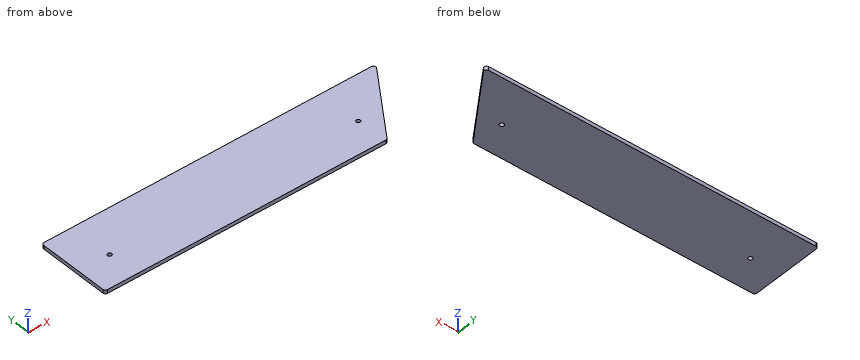
Autodesk Inventor part; units mm, degrees
ref_plane "YZ Plane" through (0, 0, 0) normal (1, 0, 0) x (0, 1, 0)
ref_plane "XZ Plane" through (0, 0, 0) normal (0, 1, 0) x (-1, 0, 0)
ref_plane "XY Plane" through (0, 0, 0) normal (0, 0, 1) x (1, 0, 0)
sketch "Sketch1" plane through (0, 0, 0) normal (0, 0, 1) x (1, 0, 0)
  line L0 (-134.5, -30) -> (134.5, -30)
  line L1 (134.5, -30) -> (134.5, 30)
  line L2 (134.5, 30) -> (-134.5, 30)
  line L3 (-134.5, 30) -> (-134.5, -30)
  line L4 (-134.5, -30) -> (134.5, 30) construction
  line L5 (134.5, -30) -> (-134.5, 30) construction
  line L6 (134.5, 30) -> (92.4875, -30)
  point P0 (0, 0)
  dimension "d0" = 269
  dimension "d1" = 60
  dimension "d2" = 55
extrude "Extrusion1" add sketch "Sketch1" along normal blind 3 contours L3 L2 L6 L0
sketch "Sketch2" plane through (0, 0, 3) normal (0, 0, 1) x (1, 0, 0)
  circle A0 centre (-109.5, -5) radius 1.65
  line L0 (-134.5, -30) -> (92.4875, -30)
  line L1 (-134.5, 30) -> (-134.5, -30)
  line L2 (-109.5, -5) -> (151.1099, -5) construction
  circle A1 centre (90.5, -5) radius 1.65
  point P0 (0, 0)
  dimension "d5" = 25
  dimension "d6" = 3.3
  dimension "d7" = 25
  dimension "d8" = 225
  dimension "d9" = 3.3
extrude "Extrusion2" cut sketch "Sketch2" against normal through all
fillet "Fillet1" radius 2 4 edges at (-134.5, 30, 1.5) (-134.5, -30, 1.5) (92.4875, -30, 1.5) (134.5, 30, 1.5)
sketch "Sketch3" plane through (0, 0, 3) normal (0, 0, 1) x (1, 0, 0)
  arc A0 (132.2963, 26.8528) -> (130.658, 30) centre (130.658, 28) ccw
  line L0 (130.658, 30) -> (-132.5, 30)
  arc A1 (-132.5, 30) -> (-134.5, 28) centre (-132.5, 28) ccw
  line L1 (-134.5, 28) -> (-134.5, -28)
  arc A2 (-134.5, -28) -> (-132.5, -30) centre (-132.5, -28) ccw
  line L2 (-132.5, -30) -> (91.4464, -30)
  arc A3 (91.4464, -30) -> (93.0847, -29.1472) centre (91.4464, -28) ccw
  line L3 (93.0847, -29.1472) -> (132.2963, 26.8528)
  circle A4 centre (90.5, -5) radius 1.65
  circle A5 centre (-109.5, -5) radius 1.65
  point P0 (0, 0)
equation "\"d9\" = d6"
properties part number "UpperAcrylicSheetSide"
The listing builds one solid part. Answer for the finished solid, in the listing's coordinates (mm). Coordinates: 2 decimals unless noted, no trailing zeros. Loops run counter-clockwise (first coordinate to the right, second up) from the corner with the lowest first, then second, coordinate; pieces in that order, holes last. Notation, with made-up numbers: (11, 26.5) -> (47, 26.5) arc R20 ccw to (47, 41.5) -> close; hole circle Ø3 at (-30.5, 43). An arc over 180 degrees is marked (long way). Answer in a Markdown table with one row per item. Add a question column.
1. The part is cut by section B-B, the plane y = -13. Write down the section's boundary in (x, z).
2. The part is cut by section C-C, the plane y = 14. Write down the section's boundary in (x, z).
3. A flat-ended cylindrical pin translates along its axis: P1, Ø1, axis at x = 97, z = 1, coming from the -Y side. Find the tip coordinate at first contact, or state that the pin passes through.
4. The part is cut by section A-A, the plane z = 1.3. Write down the section's boundary in (x, y), then the cut area to 3 significant figures.
5. Consider line 1 (Y direction, x = -109.5, z = 0.65); line 2 (X direction, y = -24.5, z = 0.5); line 3 (X direction, y = 8.5, z = 1.1). Determine where each line is inside the solid, lowest interval first. Write a range as [from, to].
Answer below:
| question | item | result |
|---|---|---|
| 1 | outline | (-134.5, 0) -> (104.39, 0) -> (104.39, 3) -> (-134.5, 3) -> close |
| 2 | outline | (-134.5, 0) -> (123.3, 0) -> (123.3, 3) -> (-134.5, 3) -> close |
| 3 | P1 | y = -24.27 |
| 4 | outline | (-134.5, -28) arc R2 ccw to (-132.5, -30) -> (91.45, -30) arc R2 ccw to (93.08, -29.15) -> (132.3, 26.85) arc R2 ccw to (130.66, 30) -> (-132.5, 30) arc R2 ccw to (-134.5, 28) -> close; hole circle Ø3.3 at (-109.5, -5); hole circle Ø3.3 at (90.5, -5) |
| 4 | area | 14,900 mm2 |
| 5 | line 1 | [-30, -6.65], [-3.35, 30] |
| 5 | line 2 | [-134.5, 96.34] |
| 5 | line 3 | [-134.5, 119.45] |
